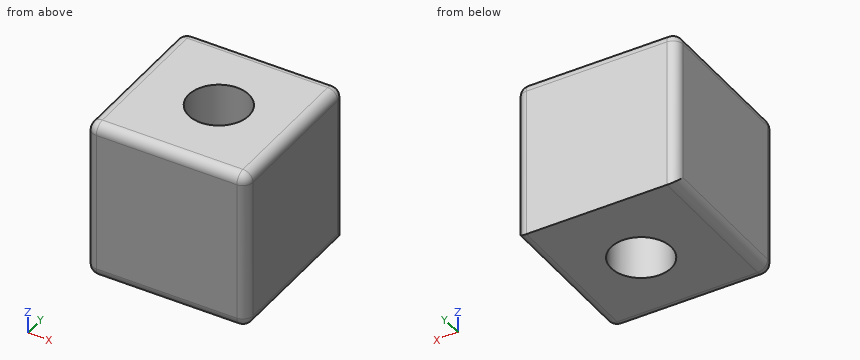
```python
from build123d import *

# Parameters (mm, degrees)
F0_W     = 80
F0_H     = 80
F1_DEPTH = 40
F2_R     = 5
F3_R     = 15
F4_DEPTH = 80.001


with BuildPart() as f1:
    # F0 (on Top) → F1 (new body, symmetric)
    with BuildSketch(Plane.XY):
        Rectangle(F0_W, F0_H)
    extrude(amount=F1_DEPTH, both=True)

    # F2
    f2_edges = [f1.edges().sort_by_distance(p)[0] for p in [
        (-40, 0, 40),
        (-40, 0, -40),
        (0, 40, 40),
        (0, -40, 40),
        (-40, -40, 0),
        (-40, 40, 0),
        (40, 0, -40),
        (40, 40, 0),
        (40, -40, 0),
        (0, -40, -40),
        (40, 0, 40),
    ]]
    fillet(f2_edges, radius=F2_R)

    # F3 (on face) → F4 (cut, through all)
    with BuildSketch(Plane.XY.offset(40)):
        with Locations((1.912538, 0)):
            Circle(F3_R)
    extrude(amount=-F4_DEPTH, mode=Mode.SUBTRACT)


solid = f1.part
```
The model under review builds one solid part; all positions refer to its coordinate system, in mm. Give positions to 0.01 mm unless a question says otherwise; leave off trailing zeros. Loops run counter-clockwise (first coordinate to the right, second up) from the corner with the lowest first, then second, coordinate; pieces in that order, holes last. Notation, with made-up numbers: (39.5, 89) - (77.5, 89) arc R13 ccw to (77.5, 107) - close; hole circle Ø7 at (62, 82.5). An arc over 180 degrees is marked (long way). Answer as a JSON object with one key per item and string values.
Q1. Add section B-B on x = 13.5. State the section outline as (y, z) points, plus the area to 3 significant figures.
Worked out:
{"outline": "(-40, -35) arc R5 ccw to (-35, -40) - (-9.53, -40) - (-9.53, 40) - (-35, 40) arc R5 ccw to (-40, 35) - close; (9.53, -40) - (40, -40) - (40, 35) arc R5 ccw to (35, 40) - (9.53, 40) - close", "area": "4,860 mm^2"}
Q2. Add section A-A on y = 0. State the section outline as (x, z) points, plus the area to 3 significant figures.
Worked out:
{"outline": "(-40, -35) arc R5 ccw to (-35, -40) - (-13.09, -40) - (-13.09, 40) - (-35, 40) arc R5 ccw to (-40, 35) - close; (16.91, -40) - (35, -40) arc R5 ccw to (40, -35) - (40, 35) arc R5 ccw to (35, 40) - (16.91, 40) - close", "area": "3,980 mm^2"}
Q3. To check wall thickness, follow line 1 along X through (y, z) = (-6.5, -9); line 2 along Y through (x, z) = (-5, 13.5); line 3 along X through (y, z) = (11.5, 1). State the ranges of each line that lie inside material, in increasing order.
Worked out:
{"line 1": "x = -40 to -11.61, 15.43 to 40", "line 2": "y = -40 to -13.31, 13.31 to 40", "line 3": "x = -40 to -7.72, 11.54 to 40"}
Q4. Add section D-D on y = -8. State the section outline as (x, z) points, plus the area to 3 significant figures.
Worked out:
{"outline": "(-40, -35) arc R5 ccw to (-35, -40) - (-10.78, -40) - (-10.78, 40) - (-35, 40) arc R5 ccw to (-40, 35) - close; (14.6, -40) - (35, -40) arc R5 ccw to (40, -35) - (40, 35) arc R5 ccw to (35, 40) - (14.6, 40) - close", "area": "4,350 mm^2"}
Q5. Add section C-C on z = 8. State the section outline as (x, y) points.
Worked out:
{"outline": "(-40, -35) arc R5 ccw to (-35, -40) - (35, -40) arc R5 ccw to (40, -35) - (40, 35) arc R5 ccw to (35, 40) - (-35, 40) arc R5 ccw to (-40, 35) - close; hole circle Ø30 at (1.91, 0)"}
